from build123d import *

# Parameters (mm, degrees)
F0_W     = 228.6
F0_H     = 254
F1_DEPTH = 939.8
F2_W     = 177.8
F2_H     = 889
F3_DEPTH = 6.35
F4_W     = 203.2
F4_H     = 889
F5_DEPTH = 6.35
F6_W     = 177.8
F6_H     = 889
F7_DEPTH = 6.35
F8_W     = 203.2
F8_H     = 889
F9_DEPTH = 6.35


with BuildPart() as f1:
    # F0 (on Top) → F1 (new body)
    with BuildSketch(Plane.XY):
        Rectangle(F0_W, F0_H)
    extrude(amount=F1_DEPTH)

    # F2 (on face) → F3 (cut)
    with BuildSketch(Plane.XZ.offset(127)):
        with Locations((0, 469.9)):
            Rectangle(F2_W, F2_H)
    extrude(amount=-F3_DEPTH, mode=Mode.SUBTRACT)

    # F4 (on face) → F5 (cut)
    with BuildSketch(Plane.YZ.offset(114.3)):
        with Locations((0, 469.9)):
            Rectangle(F4_W, F4_H)
    extrude(amount=-F5_DEPTH, mode=Mode.SUBTRACT)

    # F6 (on face) → F7 (cut)
    with BuildSketch(Plane(origin=(0, 127, 0), x_dir=(-1, 0, 0), z_dir=(0, 1, 0))):
        with Locations((0, 469.9)):
            Rectangle(F6_W, F6_H)
    extrude(amount=-F7_DEPTH, mode=Mode.SUBTRACT)

    # F8 (on face) → F9 (cut)
    with BuildSketch(Plane(origin=(-114.3, 0, 0), x_dir=(0, -1, 0), z_dir=(-1, 0, 0))):
        with Locations((0, 469.9)):
            Rectangle(F8_W, F8_H)
    extrude(amount=-F9_DEPTH, mode=Mode.SUBTRACT)


solid = f1.part
Geometry: final body of the model. Coordinates: model frame, mm. A direction names the side the tool comes from. Coordinates: 2 decimals unless noted, no trailing zeros. Order: outer loops, then holes, each group sorted by start corner. A loop starts at its lowest first (then second) coordinate and runs counter-clockwise, first axis right, second up. Notation, with made-up numbers: M 49,-19.75 L 80,-19.75 A21 cw 80,18.25 Z; hole C 81.5,83 d8. An arc over 180 degrees is marked long. One line per question, with ' | ' between items. Start each with the question number.
Item 1: Cut plane A-A, the plane y = 61. Return the cut outline in (x, z), then the cut area to 3 significant figures.
Item 2: Pin query (flat end, axial travel): pin 1 Ø8 at (x, z) = (77.5, 261.5) entering from +Y; pin 2 Ø12 at (y, z) = (13, 415.5) entering from +X; pin 3 Ø1 at (x, z) = (-45, 547.5) entering from -Y. Return the tip coordinate at first contact, or that it passes through.
Item 3: Set-up query: faces 1 (the flat face through (114.3, -104, 433)), 2 (the flat face through (-114.3, -104, 433)), 3 (the flat face through (1, 120.65, 476)), 4 (the flat face through (-1, -120.65, 476)), 5 (the flat face through (-107.95, 1, 476)). Return all of +Z, -Z, +X, -X, +Y, -Y with unobstructed straight access to the full face (end or side cutting, diameter ignored); none if empty.
Item 4: Ray query, probe 1 along Y at (x, z) = (-0.5, 400); probe 2 along X at (y, z) = (31, 836). Return the intervals inside material, ascending. Write a range as [from, to].
Item 5: Draft query along Y for faces 6 (the flat face through (-2, 2, 939.8)), 7 (the flat face through (107.95, -1, 476)), 8 (the flat face through (-94, 127, 433)). Return one class per face: released by +Y, released by -Y, zero draft, split by the parting line, or undercut.
Item 6: Cut plane C-C, the plane x = -22. Return the cut outline in (y, z).
Item 7: Cut plane B-B, the plane z = 772.5. Return the cut outline in (x, y), then the cut area to 3 significant figures.
A:
1) outline: M -114.3,0 L 114.3,0 L 114.3,25.4 L 107.95,25.4 L 107.95,914.4 L 114.3,914.4 L 114.3,939.8 L -114.3,939.8 L -114.3,914.4 L -107.95,914.4 L -107.95,25.4 L -114.3,25.4 Z | area: 204,000 mm2
2) pin 1: stops at y = 120.65 | pin 2: stops at x = 107.95 | pin 3: stops at y = -120.65
3) face 1: +Z, -Z, +X, +Y, -Y | face 2: +Z, -Z, -X, +Y, -Y | face 3: +Y | face 4: -Y | face 5: -X
4) probe 1: y = [-120.65, 120.65] | probe 2: x = [-107.95, 107.95]
5) face 6: zero draft | face 7: undercut | face 8: released by +Y
6) outline: M -127,0 L 127,0 L 127,25.4 L 120.65,25.4 L 120.65,914.4 L 127,914.4 L 127,939.8 L -127,939.8 L -127,914.4 L -120.65,914.4 L -120.65,25.4 L -127,25.4 Z
7) outline: M -114.3,-127 L -88.9,-127 L -88.9,-120.65 L 88.9,-120.65 L 88.9,-127 L 114.3,-127 L 114.3,-101.6 L 107.95,-101.6 L 107.95,101.6 L 114.3,101.6 L 114.3,127 L 88.9,127 L 88.9,120.65 L -88.9,120.65 L -88.9,127 L -114.3,127 L -114.3,101.6 L -107.95,101.6 L -107.95,-101.6 L -114.3,-101.6 Z | area: 53,200 mm2
